```python
from build123d import *

# Parameters (mm, degrees)
SKETCH_1_R      = 4.25
SKETCH_1_R_2    = 2.08
SKETCH_1_R_3    = 2
EXTRUDE_1_DEPTH = 4


with BuildPart() as part:
    # 草图1 → 凸台-拉伸1 (new body)
    with BuildSketch(Plane.XY):
        with BuildLine():
            Line((-1, 20), (99.064295006, 20))
            ThreePointArc((99.064295006, 20), (119.064295006, 0), (99.064295006, -20))
            Line((99.064295006, -20), (10.014533743, -20))
            Line((10.014533743, -20), (3, -30))
            ThreePointArc((3, -30), (-1, -34), (-5, -30))
            Line((-5, -30), (-17.208156126, -11.717323713))
            ThreePointArc((-17.208156126, -11.717323713), (-18.809358134, 9.10092099), (-1, 20))
        make_face()
        with Locations((-1, 0)):
            Circle(SKETCH_1_R, mode=Mode.SUBTRACT)
        with Locations((99.064295006, 0)):
            Circle(SKETCH_1_R, mode=Mode.SUBTRACT)
        with Locations((112.594295006, 0)):
            Circle(SKETCH_1_R_2, mode=Mode.SUBTRACT)
        with Locations((92.299295006, -11.717323713)):
            Circle(SKETCH_1_R_2, mode=Mode.SUBTRACT)
        with Locations((92.299295006, 11.717323713)):
            Circle(SKETCH_1_R_2, mode=Mode.SUBTRACT)
        with Locations((-1, -30)):
            Circle(SKETCH_1_R_3, mode=Mode.SUBTRACT)
        with BuildLine():
            Line((23.78352134, 10.95385289), (60.46647866, 10.95385289))
            ThreePointArc((60.46647866, 10.95385289), (71.420331549, 0), (60.46647866, -10.95385289))
            Line((60.46647866, -10.95385289), (23.78352134, -10.95385289))
            ThreePointArc((23.78352134, -10.95385289), (12.829668451, 0), (23.78352134, 10.95385289))
        make_face(mode=Mode.SUBTRACT)
    extrude(amount=EXTRUDE_1_DEPTH)


solid = part.part
```
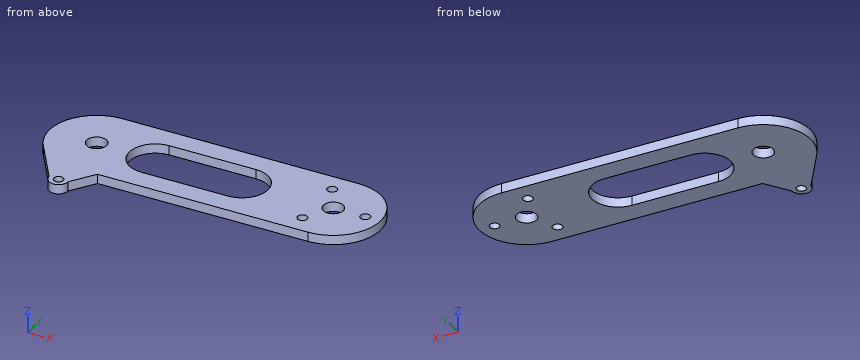
Here's how the part is built. I have some questions about the finished solid (model axes, mm). Round coordinates to 2 decimals unless told otherwise and drop trailing zeros. Write each loop counter-clockwise with the first axis right and the second up, starting at its lowest first coordinate (ties: lowest second). Pieces come first, ordered by that corner, then holes.
Q1. Please list where these lines run through material, in increasing order: probe 1 along Y at (x, z) = (-1, 1.6); probe 2 along Y at (x, z) = (24, 0.8); probe 3 along X at (y, z) = (11, 3.5).
Q2. If we section it at B-B on y = 0: Write out the boundary of the cut face in (x, z), plus the area to 3 significant figures.
Q3. If we section it at A-A on x = 45: Write out the boundary of the cut face in (y, z), plus the area to 3 significant figures.
Q4. If we section it at C-C on z = 1.3: Write out the boundary of the cut face in (x, y).
Q5. If we section it at D-D on x = 64.5: Write out the boundary of the cut face in (y, z).
Answer below:
1. probe 1: y = -34 to -32, -28 to -4.25, 4.25 to 20
1. probe 2: y = -20 to -10.95, 10.95 to 20
1. probe 3: x = -17.7 to 90.35, 94.25 to 115.77
2. outline: (-21, 0) - (-5.25, 0) - (-5.25, 4) - (-21, 4) - close; (3.25, 0) - (12.83, 0) - (12.83, 4) - (3.25, 4) - close; (71.42, 0) - (94.81, 0) - (94.81, 4) - (71.42, 4) - close; (103.31, 0) - (110.51, 0) - (110.51, 4) - (103.31, 4) - close; (114.67, 0) - (119.06, 0) - (119.06, 4) - (114.67, 4) - close
2. area: 241 mm2
3. outline: (-20, 0) - (-10.95, 0) - (-10.95, 4) - (-20, 4) - close; (10.95, 0) - (20, 0) - (20, 4) - (10.95, 4) - close
3. area: 72.4 mm2
4. outline: (-17.21, -11.72) - (-5, -30) arc R4 ccw to (3, -30) - (10.01, -20) - (99.06, -20) arc R20 ccw to (99.06, 20) - (-1, 20) arc R20 ccw to start; hole circle Ø8.5 at (-1, 0); hole circle Ø4 at (-1, -30); hole (23.78, -10.95) - (60.47, -10.95) arc R10.95 ccw to (60.47, 10.95) - (23.78, 10.95) arc R10.95 ccw to start; hole circle Ø4.16 at (92.3, -11.72); hole circle Ø4.16 at (92.3, 11.72); hole circle Ø8.5 at (99.06, 0); hole circle Ø4.16 at (112.59, 0)
5. outline: (-20, 0) - (-10.18, 0) - (-10.18, 4) - (-20, 4) - close; (10.18, 0) - (20, 0) - (20, 4) - (10.18, 4) - close
